```python
from build123d import *

# Parameters (mm, degrees)
SKETCH_R     = 2.8
PAD_DEPTH    = 3
SKETCH001_R  = 1.45
PAD001_DEPTH = 12
POCKET_DEPTH = 2
CHAMFER_SIZE = 0.25


with BuildPart() as part:
    # Sketch → Pad (new body)
    with BuildSketch(Plane.XY):
        Circle(SKETCH_R)
    extrude(amount=PAD_DEPTH)

    # Sketch001 (on Face3 of Pad) → Pad001 (join)
    with BuildSketch(Plane.XY.offset(3)):
        Circle(SKETCH001_R)
    extrude(amount=PAD001_DEPTH)

    # Sketch002 (on Face2 of Pad001) → Pocket (cut)
    with BuildSketch(Plane(origin=(0, 0, 0), x_dir=(1, 0, 0), z_dir=(0, 0, -1))):
        Polygon((1.259542, 0.814588), (-0.075682, 1.49809), (-1.335225, 0.683502), (-1.259542, -0.814588), (0.075682, -1.49809), (1.335225, -0.683502), align=None)
    extrude(amount=-POCKET_DEPTH, mode=Mode.SUBTRACT)

    # Chamfer
    chamfer_edges = [part.edges().sort_by_distance(p)[0] for p in [
        (-2.8, 0, 3),
        (-2.8, 0, 0),
        (1.297384, -0.065543, 0),
        (0.705454, 1.090796, 0),
        (-0.59193, 1.156339, 0),
        (-1.297384, 0.065543, 0),
        (-0.705454, -1.090796, 0),
        (0.59193, -1.156339, 0),
        (-1.45, 0, 15),
    ]]
    chamfer(chamfer_edges, length=CHAMFER_SIZE)


solid = part.part
```
Model file for the job. Use its own axes, mm. A direction names the side the tool comes from. Give positions to 0.01 mm unless a question says otherwise; leave off trailing zeros. Loops run counter-clockwise (first coordinate to the right, second up) from the corner with the lowest first, then second, coordinate; pieces in that order, holes last. Notation, with made-up numbers: (76.5, 47.25) -> (82.5, 47.25) arc R28 ccw to (82.5, 70.25) -> close; hole circle Ø10 at (-15.5, -11). An arc over 180 degrees is marked (long way). Write each question's results on one line, items separated by ' | '.
(1) Cut at B-B on y = 0. List the corners of the cut face in (x, z).
Geometry results:
outline: (-2.8, 0.25) -> (-2.55, 0) -> (-1.55, 0) -> (-1.3, 0.25) -> (-1.3, 2) -> (1.3, 2) -> (1.3, 0.25) -> (1.55, 0) -> (2.55, 0) -> (2.8, 0.25) -> (2.8, 2.75) -> (2.55, 3) -> (1.45, 3) -> (1.45, 14.75) -> (1.2, 15) -> (-1.2, 15) -> (-1.45, 14.75) -> (-1.45, 3) -> (-2.55, 3) -> (-2.8, 2.75) -> close
(2) Cut at A-A on z = 5.5. List the corners of the cut face in (x, y), and give its area (3 significant figures).
Geometry results:
outline: circle Ø2.9 at (0, 0) | area: 6.61 mm²
(3) Tool access for faces 4 (the flat face through (-0.6, 1.15, 1.11)), 5 (the cylindrical face through (-2.8, 0.1, 1.5)), 6 (the flat face through (0, -2, 3)): list every direction of +Z, -Z, +X, -X, +Y, -Y with a clear straight run to the whole face (end or side of a thin tool).
Geometry results:
face 4: -Z | face 5: +Z, -Z | face 6: +Z
(4) Pull direction X, two halves, no side cores. Call faces 1 (the flat face through (-0.76, -1.2, 0.13)), 2 (the flat face through (2, 0, 0)), 3 (the cylindrical face through (-1.45, 0.06, 8.79)): released by +X, released by -X, zero draft, split by the parting line, or undercut.
Geometry results:
face 1: undercut | face 2: zero draft | face 3: split by the parting line
(5) Flat gauge pins, fed straight in: pin 1 Ø3 at (x, y) = (-0.5, 2) entering from +Z; pin 2 Ø0.8 at (x, y) = (0, 0.5) entering from -Z; pin 3 Ø3 at (y, z) = (0, 12.5) entering from +X; pin 4 Ø1.5 at (x, y) = (2, -2) entering from +Z. Where does each tip first touch, or does it go through?
Geometry results:
pin 1: stops at z = 15 | pin 2: stops at z = 2 | pin 3: stops at x = 1.45 | pin 4: stops at z = 3
(6) Probe line 1 along Z through (x, y) = (0.9, -0.2); line 2 along Z through (x, y) = (1.75, 0.55); line 3 along X through (y, z) = (-1.15, 5.5). List the from-to ranges inside material, lowest first.
Geometry results:
line 1: z = 2 to 15 | line 2: z = 0 to 3 | line 3: x = -0.88 to 0.88
